```python
from build123d import *

# Parameters (mm, degrees)
F0_R     = 5
F1_DEPTH = 10
F2_R     = 4
F3_T     = -1
F5_DEPTH = 25


with BuildPart() as f1:
    # F0 (on Top) → F1 (new body)
    with BuildSketch(Plane.XY):
        Circle(F0_R)
    extrude(amount=F1_DEPTH)

    # F2
    f2_edges = [f1.edges().sort_by_distance(p)[0] for p in [
        (-5, 0, 10),
    ]]
    fillet(f2_edges, radius=F2_R)

    # F3
    f3_openings = [f1.faces().sort_by_distance(p)[0] for p in [
        (0, 0, 0),
    ]]
    offset(amount=F3_T, openings=f3_openings)

    # F4 (on Front) → F5 (cut)
    with BuildSketch(Plane.XZ):
        Polygon((3.3, 4.67722), (0, 4.67722), (-3.3, 4.67722), (-3.3, 3.92722), (-0.75, 3.92722), (-0.75, 0.911284), (0.75, 0.911284), (0.75, 3.92722), (3.3, 3.92722), align=None)
    extrude(amount=F5_DEPTH, mode=Mode.SUBTRACT)


solid = f1.part
```
The listing builds one solid part. Answer for the finished solid, in the listing's coordinates (mm). A direction names the side the tool comes from. Give positions to 0.01 mm unless a question says otherwise; leave off trailing zeros. Order: outer loops, then holes, each group sorted by start corner. A loop starts at its lowest first (then second) coordinate and runs counter-clockwise, first axis right, second up.
1) Consider line 1 along Y through (x, z) = (0, 1.55); line 2 along Y through (x, z) = (0.5, 5.25); line 3 along X through (y, z) = (-3, 6.5). Determine where each line is inside the solid, lowest interval first.
Reported:
line 1: y = 4 to 5
line 2: y = -4.97 to -3.97, 3.97 to 4.97
line 3: x = -3.96 to -2.58, 2.58 to 3.96
2) Find section A-A on z = 3.75. Write down the section's boundary in (x, y).
Reported:
outline: (-0.75, -4.94) - (-0.75, -3.93) arc R4 cw (long way) to (0.75, -3.93) - (0.75, -4.94) arc R5 ccw (long way) to start
3) For faces 4 (the face through (0, 0, 9)), 5 (the face through (0, -4.5, 0.911)), determine the directions among +Z, -Z, +X, -X, +Y, -Y from which every point of the face is accessible in a straight line to the end or side of a thin tool.
Reported:
face 4: -Z
face 5: -Y
4) Given P1, Ø2, axis at x = 2, z = 7.5, coming from the -Y side; P2, Ø2, axis at x = -3, y = 2, coming from the +Z side; P3, Ø1.6, axis at x = -0.5, y = 0.5, coming from the -Z side, each flat-ended and moving along its own axis, determine where each tip first touches the part or whether it passes through.
Reported:
P1: stops at y = -4.75
P2: stops at z = 9.66
P3: stops at z = 8.96
5) Determine the mould class of faces 1 (the face through (-0.651, 4.957, 2.958)), 2 (the face through (0.75, -4.4, 2.4)), 3 (the face through (0, 0, 10)) for opening direction X: pulls with the +X half, pulls with the -X half, needs draft (parallel to the pull), parting line crosses it, or undercut.
Reported:
face 1: parting line crosses it
face 2: undercut
face 3: needs draft
